Autodesk Fusion 360 part; units mm, degrees
sketch "Sketch1" plane through (0, 0, 0) normal (0, 1, 0) x (1, 0, 0)
  line L0 (0, 0) -> (8, 0)
  line L1 (8, 0) -> (8, -10)
  line L2 (0, -10) -> (0, 0)
  line L3 (8, -10) -> (9.0653, -13.0493)
  arc A0 (9.0653, -13.0493) -> (0, -10) centre (0, -25) ccw
extrude "Extrude1" add sketch "Sketch1" along normal blind 8
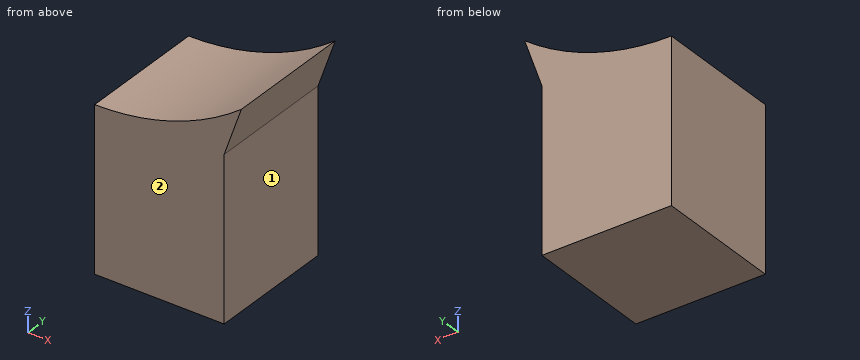
Check sheet for the modelled part. Datum: model origin and axes. Units: mm. Face numbers are marked on the shaded views. A direction names the side the tool comes from. Coordinates: 2 decimals unless noted, no trailing zeros. Write each loop counter-clockwise with the first axis right and the second up, starting at its lowest first coordinate (ties: lowest second). Pieces come first, ordered by that corner, then holes. Notation, with made-up numbers: M 18,62.5 L 38,62.5 A16 cw 38,66.5 Z; hole C -10.5,77.5 d9. An arc over 180 degrees is marked long. Write item = value, one per line. Start each with the question number.
1. Sectioned sample at B-B (z = 2.75). Record the cut outline in (x, y).
2. Tool access check on the marked faces 1 and 2. Record the directions out of +Z, -Z, +X, -X, +Y, -Y that give a thin tool (end or side, any length) a straight path to the whole face; none if there is none.
3. Sectioned sample at A-A (y = 3.5). Record the cut outline in (x, z), then the cut area to 3 significant figures.
4. Thickness scan on probe 1 along X at (y, z) = (2.25, 1.75); probe 2 along Z at (x, y) = (6, 6.75); probe 3 along Z at (x, y) = (5.25, 3). Record the ranges inside material, lowest first.
5. Go/stop test with a flat-tipped pin: pin 1 (4 mm diameter, centred on y = 6.5, z = 2.5, fed in from +X). Record where the tip stops, or that it passes through.
6. Sectioned sample at C-C (x = 8.75). Record the cut outline in (y, z), then the cut area to 3 significant figures.
The answers:
q1.outline = M 0,0 L 8,0 L 8,8 L 0,8 Z
q2.face_1 = -Z, +X, +Y, -Y
q2.face_2 = +Z, -Z, +X, -X, -Y
q3.outline = M 0,0 L 8,0 L 8,10 L 9.07,13.05 A15 cw 0,10 Z
q3.area = 87.2 mm²
q4.probe_1 = 0 to 8
q4.probe_2 = 0 to 11.25
q4.probe_3 = 0 to 10.95
q5.pin_1 = 8
q6.outline = M 0,12.15 L 8,12.15 L 8,12.82 L 0,12.82 Z
q6.area = 5.36 mm²
